The listing builds one solid part. Answer for the finished solid, in the listing's coordinates (mm). Face numbers are marked on the shaded views. Coordinates: 2 decimals unless noted, no trailing zeros. Write each loop counter-clockwise with the first axis right and the second up, starting at its lowest first coordinate (ties: lowest second). Pieces come first, ordered by that corner, then holes. Notation, with made-up numbers: M -1,62.25 L 28,62.25 A10 cw 28,70.25 Z; hole C 83,-13.75 d7. An arc over 180 degrees is marked long. Answer as CSV lines item,"result".
```python
from build123d import *

# Parameters (mm, degrees)
F1_DEPTH = 5.08
F0_R     = 2.286
F2_DEPTH = 3.556


# Not quite as in the source:
# - a fillet or chamfer that OpenCascade refuses, or shapes differently, is made with other operations: its cross-section is extruded or revolved along the edge and cut away or added


with BuildPart() as f1:
    # F0 (on Top) → F1 (new body)
    with BuildSketch(Plane.XY):
        with BuildLine():
            ThreePointArc((0, -25.4), (17.9605122421, -17.9605122421), (25.4, 0))
            ThreePointArc((25.4, 0), (17.9605122421, 17.9605122421), (0, 25.4))
            Line((0, 25.4), (0, 18.415))
            ThreePointArc((0, 18.415), (13.0213713756, 13.0213713756), (18.415, 0))
            ThreePointArc((18.415, 0), (13.0213713756, -13.0213713756), (0, -18.415))
            Line((0, -18.415), (0, -25.4))
        make_face()
        with BuildLine():
            Line((0, 18.415), (0, 25.4))
            ThreePointArc((0, 25.4), (-25.4, 0), (0, -25.4))
            Line((0, -25.4), (0, -18.415))
            ThreePointArc((0, -18.415), (-18.415, 0), (0, 18.415))
        make_face()
    extrude(amount=F1_DEPTH)

    # F0 (on Top) → F2 (join)
    with BuildSketch(Plane.XY):
        with BuildLine():
            Line((0, -18.415), (0, 18.415))
            ThreePointArc((0, 18.415), (-18.415, 0), (0, -18.415))
        make_face()
        with Locations((-7.1823259524, 0)):
            Circle(F0_R, mode=Mode.SUBTRACT)
        with BuildLine():
            ThreePointArc((18.415, 0), (13.0213713756, 13.0213713756), (0, 18.415))
            Line((0, 18.415), (0, -18.415))
            ThreePointArc((0, -18.415), (13.0213713756, -13.0213713756), (18.415, 0))
        make_face()
        with Locations((7.1823259524, 0)):
            Circle(F0_R, mode=Mode.SUBTRACT)
    extrude(amount=F2_DEPTH)

    # F3: fillet of radius 5.08 on 1 edges, made by hand

    # F3_s1 → F3_t2 (revolve, cut)
    with BuildSketch(Plane.XZ):
        with BuildLine():
            ThreePointArc((22.0428456417, 5.08), (20.0753701018, 4.6835285843), (18.415, 3.556))
            Line((18.415, 3.556), (18.415, 5.08))
            Line((18.415, 5.08), (22.0428456417, 5.08))
        make_face()
    revolve(axis=Axis((0, 0, 5.08), (0, 0, -1)), mode=Mode.SUBTRACT)


solid = f1.part
```
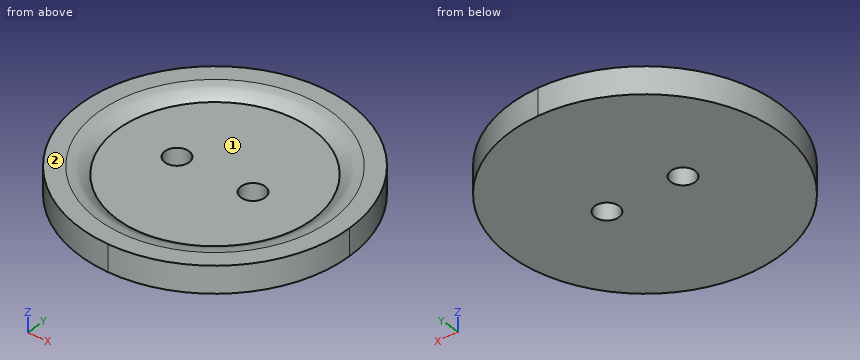
Q1. The mould has two halves that part along Y. Classify the marked faces 1 and 2: pulls with the +Y half, pulls with the -Y half, needs draft (parallel to the pull), parting line crosses it, or undercut.
Output:
face 1,"undercut"
face 2,"needs draft"
Q2. Flat-ended cylindrical pins translate along their axes: pin 1 Ø11 at (x, y) = (5.5, -4) entering from +Z; pin 2 Ø1.5 at (x, z) = (12, 2.5) entering from +Y. Find the tip coordinate at first contact, or state that the pin passes through.
Output:
pin 1,"z = 3.56"
pin 2,"y = 22.77"
Q3. Find section A-A (z = 0.75). Give the vertices of the cut face in (x, y), and give its area (3 significant figures).
Output:
outline,"C 0,0 d50.8; hole C -7.18,0 d4.57; hole C 7.18,0 d4.57"
area,"1,990 mm2"
Q4. Straight lines are drawn through the part: line 1 (Z direction, x = -5.5, y = 16); line 2 (Y direction, x = 7.5, z = 4.4); line 3 (Y direction, x = 3.5, z = 3.6). For each, find the intervals that lie inside material, in ascending order.
Output:
line 1,"0 to 3.56"
line 2,"-24.27 to -18, 18 to 24.27"
line 3,"-25.16 to -18.12, 18.12 to 25.16"
